Build history of the part. All positions in model axes, mm. Round coordinates to 2 decimals unless told otherwise and drop trailing zeros. Loops run counter-clockwise (first coordinate to the right, second up) from the corner with the lowest first, then second, coordinate; pieces in that order, holes last. Notation, with made-up numbers: (-17.5, -33.75) - (21.5, -33.75) arc R32 cw to (21.5, -5.75) - close; hole circle Ø6 at (79, -5). An arc over 180 degrees is marked (long way). Answer as CSV lines item,"result". Start each with the question number.
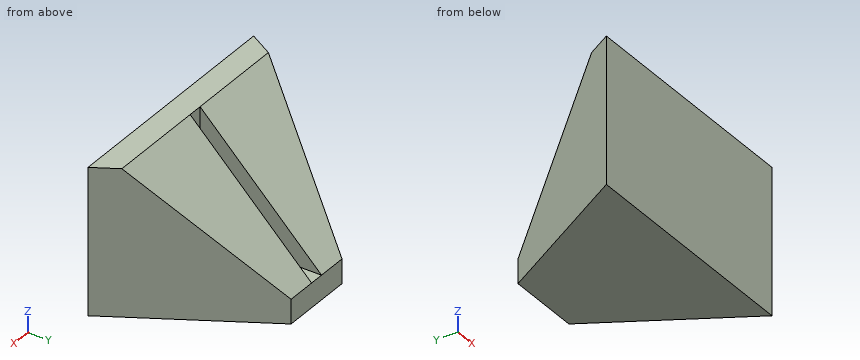
```python
from build123d import *

# Parameters (mm, degrees)
F1_DEPTH      = 5
F4_DEPTH      = 25
F5_DEPTH      = 23.1132486541
F5_DEPTH_BACK = 23.1132486541


with BuildPart() as f1:
    # F0 (on Top) → F1 (new body)
    with BuildSketch(Plane.XY):
        Polygon((7.6794919243, 21.294143835), (-7.6794919243, 21.294143835), (-25, -8.705856165), (25, -8.705856165), align=None)
    extrude(amount=F1_DEPTH)

    # F2 (on face) → F4 (join, through all)
    with BuildSketch(Plane.XY.offset(5)):
        Polygon((-1.5, -3.705856165), (-1.5, 21.294143835), (-7.6794919243, 21.294143835), (-25, -8.705856165), (25, -8.705856165), (7.6794919243, 21.294143835), (1.5, 21.294143835), (1.5, -3.705856165), align=None)
    extrude(amount=F4_DEPTH)

    # F3 (on Right) → F5 (cut, two sides)
    with BuildSketch(Plane.YZ) as f5_sk:
        Polygon((-3.705856165, 30), (21.294143835, 5), (21.294143835, 30), align=None)
    extrude(amount=-F5_DEPTH, mode=Mode.SUBTRACT)
    extrude(f5_sk.sketch, amount=F5_DEPTH_BACK, mode=Mode.SUBTRACT)


solid = f1.part
```
Q1. Wall check: probe 1 along X at (y, z) = (-3, 26); probe 2 along X at (y, z) = (0.5, 9) (3 decimals); probe 3 along Y at (x, z) = (-17, 16). Give the ranges that are in metal, low to high. Write a range as [from, to].
Q2. Band-saw the part on C-C, the plane x = 4.5. List the corners of the cut face in (y, z), then the cut area to 4 significant figures.
Q3. Pin check, flat tips, straight feed: pin 1 Ø7.5 at (y, z) = (6, 13.5) entering from +X; pin 2 Ø4 at (y, z) = (4, 15.5) entering from +X; pin 3 Ø12 at (x, z) = (-2.5, 22) entering from +Y. Stop position of each tip, or through.
Q4. Band-saw the part on A-A, the plane z = 25.5. List the corners of the cut face in (x, y).
Q5. Band-saw the part on D-D, the plane x = -0.5. List the corners of the cut face in (y, z).
Q6. Band-saw the part on B-B, the plane y = 5.5. List the corners of the cut face in (x, z).
Reported:
1,probe 1,"x = [-21.71, -1.5], [1.5, 21.71]"
1,probe 2,"x = [-19.685, -1.5], [1.5, 19.685]"
1,probe 3,"y = [-8.71, 5.15]"
2,outline,"(-8.71, 0) - (21.29, 0) - (21.29, 5) - (-3.71, 30) - (-8.71, 30) - close"
2,area,"587.5 mm2"
3,pin 1,"stops at x = 18.67"
3,pin 2,"stops at x = 18.82"
3,pin 3,"stops at y = 10.29"
4,outline,"(-25, -8.71) - (25, -8.71) - (19.52, 0.79) - (1.5, 0.79) - (1.5, -3.71) - (-1.5, -3.71) - (-1.5, 0.79) - (-19.52, 0.79) - close"
5,outline,"(-8.71, 0) - (21.29, 0) - (21.29, 5) - (-3.71, 5) - (-3.71, 30) - (-8.71, 30) - close"
6,outline,"(-16.8, 0) - (16.8, 0) - (16.8, 20.79) - (1.5, 20.79) - (1.5, 5) - (-1.5, 5) - (-1.5, 20.79) - (-16.8, 20.79) - close"
